Can you work these out from the model? Positions are in its coordinate system, mm. A direction names the side the tool comes from. Coordinates: 2 decimals unless noted, no trailing zeros. Write each loop counter-clockwise with the first axis right and the second up, starting at its lowest first coordinate (ties: lowest second). Pieces come first, ordered by that corner, then holes. Notation, with made-up numbers: (43, 86) - (49, 86) arc R22 cw to (49, 106) - close; hole circle Ø1 at (1, 48). An arc over 180 degrees is marked (long way). Use one line per item in the form item = value. Start each with the question number.
(1) If we section it at B-B on x = -40.5: Please give me the cut outline in (y, z).
(2) If we section it at D-D on z = 5: Please give me the cut outline in (x, y), then the cut area to 3 significant figures.
(3) On a 3-axis mill with a long thin cutter (end or side, diameter ignored), from which of +Z, -Z, +X, -X, +Y, -Y can I reach the whole of each face in a straight line? I mean faces 5 (the face through (-1, 0, 1)), 6 (the face through (-1.13, -35.72, -8.64)). Say none if no direction works.
(4) Thinking about a two-plate mould opening in Z: for faces 1 (the face through (68.48, -35.72, 21.57)), 2 (the face through (0, -76.2, 2)), 3 (the face through (2, -2.54, -2)), 4 (the face through (-16.11, -34.44, -72.57)), which applies, pulls with the +Z half, pulls with the -Z half, needs draft (parallel to the pull), parting line crosses it, or undercut?
(5) If we section it at C-C on z = 46.5: Please give me the cut outline in (x, y).
(6) For pin 1 Ø3 at (x, y) = (4, -37.5) entering from +Z; pin 2 Ø3 at (x, y) = (-59, -43.5) entering from -Z; pin 3 Ø7 at (x, z) = (5, -3.5) entering from -Y; pin 4 Ø8 at (x, z) = (55, -52.5) entering from +Y, each with a flat end and sliding along its axis, tell me the tip position at first contact or that it passes through.
(7) If we section it at A-A on y = -27.5: Please give me the cut outline in (x, z), then the cut area to 3 significant figures.
(8) If I drill on probe 1 along Z at (x, y) = (0, -19); probe 2 along Y at (x, z) = (-5.5, 26); probe 3 along Z at (x, y) = (-56, -54), over which ranges is the centre line in solid material (lowest first)? Write a range as from..to.
```python
from build123d import *

# Parameters (mm, degrees)
F0_R     = 74.3348604036
F1_DEPTH = 69.85
F2_T     = -2.54
F3_R     = 11.2538360461
F4_DEPTH = 67.31
F5_T     = -2.54
F6_R     = 2.3281724299
F7_DEPTH = 73.66
F9_DEPTH = 2.54


# Not quite as in the source:
# - a shell that OpenCascade refuses in one call is made with other operations: the cavity is built on its own and cut out


with BuildPart() as f1:
    # F0 (on Front) → F1 (new body)
    with BuildSketch(Plane.XZ):
        Circle(F0_R)
    extrude(amount=F1_DEPTH)

    # F2
    f2_openings = [f1.faces().sort_by_distance(p)[0] for p in [
        (0, -69.85, 0),
    ]]
    offset(amount=F2_T, openings=f2_openings)

    # F3 (on face) → F4 (join)
    with BuildSketch(Plane.XZ.offset(2.54)):
        Circle(F3_R)
    extrude(amount=F4_DEPTH)

    # F5: a shell. OpenCascade refuses it in one call, so the cavity is built on its own and cut out:
    # the body offset inwards by the wall thickness, plus a prism from it out through each open face.
    f5_core = offset(f1.part, amount=F5_T, kind=Kind.INTERSECTION, mode=Mode.PRIVATE)
    f5_exits = [f5_core.faces().sort_by_distance(p)[0] for p in [
        (0, -67.31, 0),
    ]]
    add(f5_core, mode=Mode.SUBTRACT)
    extrude(f5_exits, amount=-F5_T, mode=Mode.SUBTRACT)

    # F6 (on face) → F7 (join)
    with BuildSketch(Plane.XZ.offset(2.54)):
        Circle(F6_R)
    extrude(amount=F7_DEPTH)

    # F8 (on face) → F9 (join)
    with BuildSketch(Plane.XZ.offset(76.2)):
        with BuildLine():
            Line((1.6746039799, 1.552517079), (-1.7349575161, 1.552517079))
            Line((-1.7349575161, 1.552517079), (-1.7349575161, -1.552517079))
            ThreePointArc((-1.7349575161, -1.552517079), (-1.7050897064, -1.5852621097), (-1.6746039799, -1.6174326489))
            Line((-1.6746039799, -1.6174326489), (1.6746039799, -1.6174326489))
            Line((1.6746039799, -1.6174326489), (1.6746039799, 1.552517079))
        make_face()
    extrude(amount=F9_DEPTH)


solid = f1.part
```
Reported:
q1.outline = (-69.85, -62.33) - (0, -62.33) - (0, 62.33) - (-69.85, 62.33) - (-69.85, 59.28) - (-2.54, 59.28) - (-2.54, -59.28) - (-69.85, -59.28) - close
q2.outline = (-74.17, -69.85) - (-71.62, -69.85) - (-71.62, -2.54) - (-10.08, -2.54) - (-10.08, -69.85) - (-7.14, -69.85) - (-7.14, -2.54) - (7.14, -2.54) - (7.14, -69.85) - (10.08, -69.85) - (10.08, -2.54) - (71.62, -2.54) - (71.62, -69.85) - (74.17, -69.85) - (74.17, 0) - (-74.17, 0) - close
q2.area = 1,120 mm2
q3.face_5 = +Z, -Z, +X, -X, +Y
q3.face_6 = -Y
q4.face_1 = undercut
q4.face_2 = needs draft
q4.face_3 = undercut
q4.face_4 = parting line crosses it
q5.outline = (-58, -69.85) - (-54.7, -69.85) - (-54.7, -2.54) - (54.7, -2.54) - (54.7, -69.85) - (58, -69.85) - (58, 0) - (-58, 0) - close
q6.pin_1 = 74.29
q6.pin_2 = -47.11
q6.pin_3 = -69.85
q6.pin_4 = 0
q7.outline = circle Ø148.67 at (0, 0); circle Ø22.51 at (0, 0); circle Ø4.66 at (0, 0); hole circle Ø143.59 at (0, 0); hole circle Ø17.43 at (0, 0)
q7.area = 1,340 mm2
q8.probe_1 = -74.33..-71.79, -11.25..-8.71, -2.33..2.33, 8.71..11.25, 71.79..74.33
q8.probe_2 = -2.54..0
q8.probe_3 = -48.88..-44.93, 44.93..48.88
